```python
from build123d import *

# Parameters (mm, degrees)
F0_W      = 22
F0_H      = 10
F1_DEPTH  = 19
F2_W      = 19
F2_H      = 19
F3_DEPTH  = 10
F4_W      = 9
F4_H      = 5
F5_DEPTH  = 4
F7_DEPTH  = 25
F9_DEPTH  = 19
F10_DEPTH = 25
F12_DEPTH = 10
F14_DEPTH = 8
F16_DEPTH = 3


# Not quite as in the source:
# - a feature names something its author has since deleted; it is built from what else it names


with BuildPart() as f1:
    # F0 (on Right) → F1 (new body)
    with BuildSketch(Plane.YZ):
        with Locations((10.6502909437, -9.5214466426)):
            Rectangle(F0_W, F0_H)
    extrude(amount=F1_DEPTH)

    # F2 (on face) → F3 (join)
    with BuildSketch(Plane.XY.offset(-4.5214466426)):
        with Locations((9.5, -9.8497090563)):
            Rectangle(F2_W, F2_H)
    extrude(amount=-F3_DEPTH)

    # F4 (on face) → F5 (cut)
    with BuildSketch(Plane(origin=(0, 0, -14.5214466426), x_dir=(1, 0, 0), z_dir=(0, 0, -1))):
        with Locations((14.5, 8.3497090563)):
            Rectangle(F4_W, F4_H)
        with Locations((14.5, -10.6502909437)):
            Rectangle(F4_W, F4_H)
    extrude(amount=-F5_DEPTH, mode=Mode.SUBTRACT)

    # F6 (on face) → F7 (cut)
    with BuildSketch(Plane(origin=(0, 0, 0), x_dir=(0, -1, 0), z_dir=(-1, 0, 0))):
        with BuildLine():
            Line((-7.5971894228, -14.5214466426), (5.2966075354, -14.5214466426))
            ThreePointArc((5.2966075354, -14.5214466426), (-1.1502909437, -12.7714466426), (-7.5971894228, -14.5214466426))
        make_face()
        with BuildLine():
            ThreePointArc((-7.5971894228, -14.5214466426), (-7.4892397679, -36.5840063737), (11.5997090563, -25.5214466426))
            ThreePointArc((11.5997090563, -25.5214466426), (9.9122687874, -19.1824978184), (5.2966075354, -14.5214466426))
            Line((5.2966075354, -14.5214466426), (-7.5971894228, -14.5214466426))
        make_face()
    extrude(amount=-F7_DEPTH, mode=Mode.SUBTRACT)

    # F8 (on face) → F9 (join)
    with BuildSketch(Plane(origin=(0, 0, 0), x_dir=(0, -1, 0), z_dir=(-1, 0, 0))):
        with BuildLine():
            ThreePointArc((19.3497090563, -7.2717528529), (78.9260517523, -115.1245254627), (173.8108090563, -36.5214466426))
            ThreePointArc((173.8108090563, -36.5214466426), (110.1555805515, 41.7910583919), (20.489597937, -4.5214466426))
            Line((20.489597937, -4.5214466426), (33.1326909363, -4.5214466426))
            Line((33.1326909363, -4.5214466426), (33.1326909363, -14.5214466426))
            Line((33.1326909363, -14.5214466426), (19.3497090563, -14.5214466426))
            Line((19.3497090563, -14.5214466426), (19.3497090563, -7.2717528529))
        make_face()
        with BuildLine():
            ThreePointArc((19.3497090563, -7.2717528529), (19.9068584447, -5.8912967246), (20.489597937, -4.5214466426))
            Line((20.489597937, -4.5214466426), (19.3497090563, -4.5214466426))
            Line((19.3497090563, -4.5214466426), (19.3497090563, -7.2717528529))
        make_face()
    extrude(amount=-F9_DEPTH)

    # F8 (on face) → F10 (cut)
    with BuildSketch(Plane(origin=(0, 0, 0), x_dir=(0, -1, 0), z_dir=(-1, 0, 0))):
        with BuildLine():
            ThreePointArc((19.3497090563, -7.2717528529), (78.9260517523, -115.1245254627), (173.8108090563, -36.5214466426))
            ThreePointArc((173.8108090563, -36.5214466426), (110.1555805515, 41.7910583919), (20.489597937, -4.5214466426))
            Line((20.489597937, -4.5214466426), (33.1326909363, -4.5214466426))
            Line((33.1326909363, -4.5214466426), (33.1326909363, -14.5214466426))
            Line((33.1326909363, -14.5214466426), (19.3497090563, -14.5214466426))
            Line((19.3497090563, -14.5214466426), (19.3497090563, -7.2717528529))
        make_face()
    extrude(amount=-F10_DEPTH, mode=Mode.SUBTRACT)

    # F11 (on face) → F12 (join)
    with BuildSketch(Plane(origin=(0, 0, 0), x_dir=(0, -1, 0), z_dir=(-1, 0, 0))):
        with BuildLine():
            ThreePointArc((-10.6762534344, -17.046864728), (-9.2359267268, -15.6632016678), (-7.5971894228, -14.5214466426))
            Line((-7.5971894228, -14.5214466426), (-21.6502909437, -14.5214466426))
            Line((-21.6502909437, -14.5214466426), (-21.6502909437, -18.9818836282))
            Line((-21.6502909437, -18.9818836282), (-10.6762534344, -17.046864728))
        make_face()
    extrude(amount=-F12_DEPTH)

    # F13 (on face) → F14 (cut)
    with BuildSketch(Plane.YZ.offset(19)):
        Polygon((1.1502909437, -4.5214466426), (-6.8497090563, -4.5214466426), (-6.8497090563, -10.5214466426), (-5.8497090563, -10.5214466426), (1.1502909437, -10.5214466426), align=None)
        Polygon((9.1502909437, -4.5214466426), (1.1502909437, -4.5214466426), (1.1502909437, -10.5214466426), (8.1502909437, -10.5214466426), (9.1502909437, -10.5214466426), align=None)
    extrude(amount=-F14_DEPTH, mode=Mode.SUBTRACT)

    # F15 (on face) → F16 (join)
    with BuildSketch(Plane.XY.offset(-4.5214466426)):
        with BuildLine():
            ThreePointArc((19, -6.3497090563), (11.5, 1.1502909437), (19, 8.6502909437))
            Line((19, 8.6502909437), (19, 9.1502909437))
            Line((19, 9.1502909437), (11, 9.1502909437))
            Line((11, 9.1502909437), (11, -6.8497090563))
            Line((11, -6.8497090563), (19, -6.8497090563))
            Line((19, -6.8497090563), (19, -6.3497090563))
        make_face()
    extrude(amount=-F16_DEPTH)


solid = f1.part
```
Verification items for the finished model (mm, model axes). A direction names the side the tool comes from. Give positions to 0.01 mm unless a question says otherwise; leave off trailing zeros. Order: outer loops, then holes, each group sorted by start corner. A loop starts at its lowest first (then second) coordinate and runs counter-clockwise, first axis right, second up. Notation, with made-up numbers: M 38,-39.75 L 60,-39.75 A31 cw 60,-13.75 Z; hole C -10.75,19 d8. An arc over 180 degrees is marked long. Return JSON: item names as keys, results as strings. Group by question number.
1) Access from +Z, -Z, +X, -X, +Y, -Y to the whole of each face (thin tool, end or side, straight path). Record for faces 5 (the face through (11.5, 1, -6)), 6 (the face through (14, 8.15, -13)), 7 (the face through (7, -12, -14.521)), 8 (the face through (15, 1, -10.521)), 9 (the face through (14, 17, -14.521)).
2) Section check C-C on y = -1.5. Record the cut outline in (x, z), and give its area (3 significant figures).
3) Scan lines: line 1 (Z direction, x = 14.25, y = -11.5); line 2 (Y direction, x = 7.5, z = -7.25); line 3 (X direction, y = -6.5, z = -10.25). Record each from-to range of solid material in increasing order.
4) Section check A-A on x = 13. Record the cut outline in (y, z).
5) Go/stop test with flat-tipped pins: pin 1 Ø1.5 at (x, y) = (16.5, 9.5) entering from -Z; pin 2 Ø3.5 at (x, z) = (13.5, -8.5) entering from -Y; pin 3 Ø1.2 at (x, z) = (12.5, -12) entering from -Y; pin 4 Ø3 at (y, z) = (5.5, -17) entering from -X. Record where each tip stops, or that it passes through.
6) Mould release check, pull along Y, two halves, no side actions. Record for faces 1 (the face through (4.93, 16.24, -18.028)), 2 (the face through (15, 9.15, -9)), 3 (the face through (9, 21.65, -10)), 4 (the face through (0, 6, -10)): pulls with the +Y half, pulls with the -Y half, needs draft (parallel to the pull), parting line crosses it, or undercut.
7) Section check D-D on x = 3.25. Record the cut outline in (y, z).
8) Section check B-B on z = -11. Record the cut outline in (x, y), and give its area (3 significant figures).
Answer block:
{
 "1": {"face 5": "+Z, +X", "face 6": "-Z, +X", "face 7": "-Z, +X, -X, -Y", "face 8": "+X", "face 9": "-Z, +X, +Y, -Y"},
 "2": {"outline": "M 0,-13.05 L 19,-13.05 L 19,-10.52 L 11,-10.52 L 11,-7.52 L 11.98,-7.52 L 11.98,-4.52 L 0,-4.52 Z", "area": "117 mm^2"},
 "3": {"line 1": "z = -14.52 to -4.52", "line 2": "y = -19.36 to 21.65", "line 3": "x = 0 to 11"},
 "4": {"outline": "M -20.49,-4.52 A80 cw -16.9,-14.52 L -10.85,-14.52 L -10.85,-10.52 L -6.85,-10.52 L -6.85,-7.52 L -3.35,-7.52 L -3.35,-4.52 Z; M -5.85,-14.52 L -5.3,-14.52 A12.75 cw 7.6,-14.52 L 8.15,-14.52 L 8.15,-10.52 L -5.85,-10.52 Z; M 5.65,-7.52 L 9.15,-7.52 L 9.15,-10.52 L 13.15,-10.52 L 13.15,-14.52 L 21.65,-14.52 L 21.65,-4.52 L 5.65,-4.52 Z"},
 "5": {"pin 1": "stops at z = -10.52", "pin 2": "stops at y = -19.56", "pin 3": "stops at y = -17.86", "pin 4": "passes through"},
 "6": {"face 1": "pulls with the -Y half", "face 2": "undercut", "face 3": "pulls with the +Y half", "face 4": "needs draft"},
 "7": {"outline": "M -20.49,-4.52 A80 cw -16.9,-14.52 L -5.3,-14.52 A12.75 cw 10.68,-17.05 L 21.65,-18.98 L 21.65,-4.52 Z"},
 "8": {"outline": "M 0,-17.99 L 19,-17.99 L 19,-10.85 L 10,-10.85 L 10,-5.85 L 19,-5.85 L 19,8.15 L 10,8.15 L 10,13.15 L 19,13.15 L 19,21.65 L 0,21.65 Z", "area": "663 mm^2"}
}
